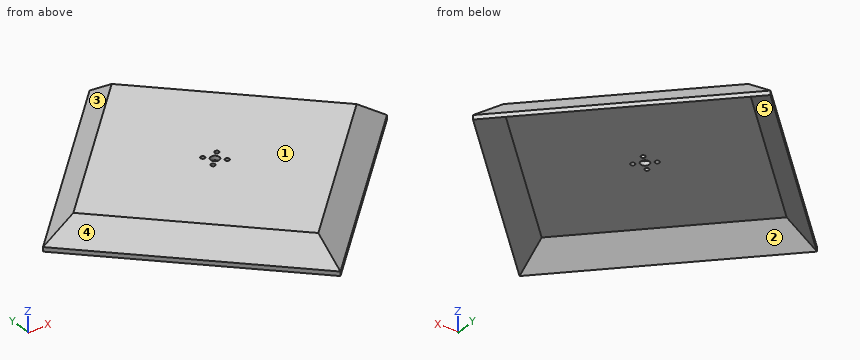
```python
from build123d import *

# Parameters (mm, degrees)
SKETCH_1_W               = 170
SKETCH_1_H               = 170
EXTRUDE_1_DEPTH          = 3
SKETCH_3_R               = 3
SKETCH_3_R_2             = 1.5
CUT_EXTRUDE_1_DEPTH      = 121.245582039
FILLET_1_R               = 2
CUT_EXTRUDE_START        = -10
CUT_EXTRUDE_2_DEPTH      = 10
CUT_EXTRUDE_START_2      = -3
CUT_EXTRUDE_3_DEPTH      = 3
EXTRUDE_4_DEPTH          = 3
EXTRUDE_5_DEPTH          = 170
PATTERN_CIRCULAR_1_COUNT = 4
CUT_EXTRUDE_4_DEPTH      = 179
PATTERN_CIRCULAR_2_COUNT = 4


with BuildPart() as part:
    # 草图1 → 凸台-拉伸1 (new body)
    with BuildSketch(Plane.XY):
        Rectangle(SKETCH_1_W, SKETCH_1_H)
    extrude(amount=EXTRUDE_1_DEPTH)

    # 草图3 → 切除-拉伸1 (cut, through all)
    with BuildSketch(Plane(origin=(0, 0, 0), x_dir=(-1, 0, 0), z_dir=(0, 0, -1))):
        Circle(SKETCH_3_R)
        with Locations((4.95, 4.95)):
            Circle(SKETCH_3_R_2)
        with Locations((-4.95, 4.95)):
            Circle(SKETCH_3_R_2)
        with Locations((-4.95, -4.95)):
            Circle(SKETCH_3_R_2)
        with Locations((4.95, -4.95)):
            Circle(SKETCH_3_R_2)
    extrude(amount=-CUT_EXTRUDE_1_DEPTH, mode=Mode.SUBTRACT)

    # 圆角1
    fillet_1_edges = [part.edges().sort_by_distance(p)[0] for p in [
        (-85, 85, 1.5),
        (85, 85, 1.5),
        (85, -85, 1.5),
        (-85, -85, 1.5),
    ]]
    fillet(fillet_1_edges, radius=FILLET_1_R)

    # 草图4 → 切除-拉伸2 (cut)
    with BuildSketch(Plane(origin=(0, 0, 0), x_dir=(-1, 0, 0), z_dir=(0, 0, -1)).offset(CUT_EXTRUDE_START)):
        with BuildLine():
            Line((-85, 35.208152802), (-60.104076401, 60.104076401))
            Line((-60.104076401, 60.104076401), (-35.208152802, 85))
            Line((-35.208152802, 85), (-83, 85))
            ThreePointArc((-83, 85), (-84.414213562, 84.414213562), (-85, 83))
            Line((-85, 83), (-85, 35.208152802))
        make_face()
        with BuildLine():
            Line((85, -35.208152802), (60.104076401, -60.104076401))
            Line((60.104076401, -60.104076401), (35.208152802, -85))
            Line((35.208152802, -85), (83, -85))
            ThreePointArc((83, -85), (84.414213562, -84.414213562), (85, -83))
            Line((85, -83), (85, -35.208152802))
        make_face()
    extrude(amount=CUT_EXTRUDE_2_DEPTH, mode=Mode.SUBTRACT)

    # 草图6 → 切除-拉伸3 (cut)
    with BuildSketch(Plane(origin=(0, 0, 0), x_dir=(-1, 0, 0), z_dir=(0, 0, -1)).offset(CUT_EXTRUDE_START_2)):
        with BuildLine():
            Line((-35.208152802, -85), (-60.104076401, -60.104076401))
            Line((-60.104076401, -60.104076401), (-85, -35.208152802))
            Line((-85, -35.208152802), (-85, -83))
            ThreePointArc((-85, -83), (-84.414213562, -84.414213562), (-83, -85))
            Line((-83, -85), (-35.208152802, -85))
        make_face()
        with BuildLine():
            Line((35.208152802, 85), (60.104076401, 60.104076401))
            Line((60.104076401, 60.104076401), (85, 35.208152802))
            Line((85, 35.208152802), (85, 83))
            ThreePointArc((85, 83), (84.414213562, 84.414213562), (83, 85))
            Line((83, 85), (35.208152802, 85))
        make_face()
    extrude(amount=CUT_EXTRUDE_3_DEPTH, mode=Mode.SUBTRACT)

    # 草图7 → 凸台-拉伸4 (add)
    with BuildSketch(Plane(origin=(0, 0, 0), x_dir=(-1, 0, 0), z_dir=(0, 0, -1))):
        Polygon((-85, 35.208152802), (-120.208152802, 0), (-85, -35.208152802), align=None)
        Polygon((0, 120.208152802), (-35.208152802, 85), (35.208152802, 85), align=None)
        Polygon((35.208152802, -85), (-35.208152802, -85), (0, -120.208152802), align=None)
        Polygon((120.208152802, 0), (85, 35.208152802), (85, -35.208152802), align=None)
    extrude(amount=-EXTRUDE_4_DEPTH)

    # 草图8 → 凸台-拉伸5 (add)
    with BuildSketch(Plane(origin=(-60.104076401, 60.104076401, 0), x_dir=(0, 0, 1), z_dir=(-0.7071067811865438, 0.7071067811865513, 0))):
        Polygon((0, 73), (-12, 85), (-15, 85), (0, 70), align=None)
    extrude_5 = extrude(amount=-EXTRUDE_5_DEPTH)

    # 阵列(圆周)1: 凸台-拉伸5 ×4 about axis
    pattern_circular_1_axis = Axis((0, 0, 0), (0, 0, 1))
    for i in range(1, PATTERN_CIRCULAR_1_COUNT):
        add(extrude_5.rotate(pattern_circular_1_axis, i * 360 / PATTERN_CIRCULAR_1_COUNT))

    # 草图9 → 切除-拉伸4 (cut)
    with BuildSketch(Plane(origin=(60.104076401, 60.104076401, 0), x_dir=(0, 0, -1), z_dir=(0.7071067811865486, 0.7071067811865465, 0))):
        Polygon((-3, 85), (12, 85), (-3, 70), align=None)
    cut_extrude_4 = extrude(amount=-CUT_EXTRUDE_4_DEPTH, mode=Mode.SUBTRACT)

    # 阵列(圆周)2: 切除-拉伸4 ×4 about axis
    pattern_circular_2_axis = Axis((0, 0, 0), (0, 0, -1))
    for i in range(1, PATTERN_CIRCULAR_2_COUNT):
        add(cut_extrude_4.rotate(pattern_circular_2_axis, i * 360 / PATTERN_CIRCULAR_2_COUNT), mode=Mode.SUBTRACT)


solid = part.part
```
Can you work these out from the model? Positions are in its coordinate system, mm. Face numbers are marked on the shaded views. A direction names the side the tool comes from. Coordinates: 2 decimals unless noted, no trailing zeros. Order: outer loops, then holes, each group sorted by start corner. A loop starts at its lowest first (then second) coordinate and runs counter-clockwise, first axis right, second up.
1. If we section it at C-C (x = 77.5): Please give me the cut outline in (y, z), then the cut area to 3 significant figures.
2. I'm going to push flat-ended pins straight in: pin 1 (5 mm diameter, centred on x = -30.5, y = 38.5, fed in from -Z); pin 2 (1.5 mm diameter, centred on x = 20.5, z = -9.5, fed in from -Y); pin 3 (1 mm diameter, centred on y = 28, z = -9, fed in from +X). Where does each tip first touch, or does it pass through?
3. I need wall thicknesses on line 1 (Y direction, x = -4.95, z = 1); line 2 (Y direction, x = 4.95, z = 1.2); line 3 (Z direction, x = -48, y = 43). Which ranges of each line are inside material? Lowest first, please.
4. For the marked faces 1 and 2, which set-ups out of +Z, -Z, +X, -X, +Y, -Y let a thin tool reach every point of the face, with its end or its side?
5. Thinking about a two-plate mould opening in Y: for the marked faces 3, 4 and 5, which applies, +Y half, -Y half, draft (parallel to the pull), parting line (faces both ways), or undercut?
6. If we section it at B-B (y = -80): Please give me the cut outline in (x, z), then the cut area to 3 significant figures.
7. If we section it at A-A (z = -9): Please give me the cut outline in (x, y).
Entries:
1. outline: (-42.71, -15) - (-21.49, 0) - (21.49, 0) - (42.71, -15) - (42.71, -12) - (21.49, 3) - (-21.49, 3) - (-42.71, -12) - close
1. area: 256 mm2
2. pin 1: stops at z = 0
2. pin 2: stops at y = -97.47
2. pin 3: stops at x = 88.83
3. line 1: y = -96.87 to -6.45, -3.45 to 3.45, 6.45 to 96.87
3. line 2: y = -96.59 to -6.45, -3.45 to 3.45, 6.45 to 96.59
3. line 3: z = 0 to 3
4. face 1: +Z, +X, -X, +Y, -Y
4. face 2: -Z
5. face 3: +Y half
5. face 4: -Y half
5. face 5: undercut
6. outline: (-40.21, -15) - (-18.99, 0) - (18.99, 0) - (40.21, -15) - (40.21, -12) - (18.99, 3) - (-18.99, 3) - (-40.21, -12) - close
6. area: 241 mm2
7. outline: (-115.97, 0) - (0, -115.97) - (115.97, 0) - (0, 115.97) - close; hole (-111.72, 0) - (0, -111.72) - (111.72, 0) - (0, 111.72) - close
